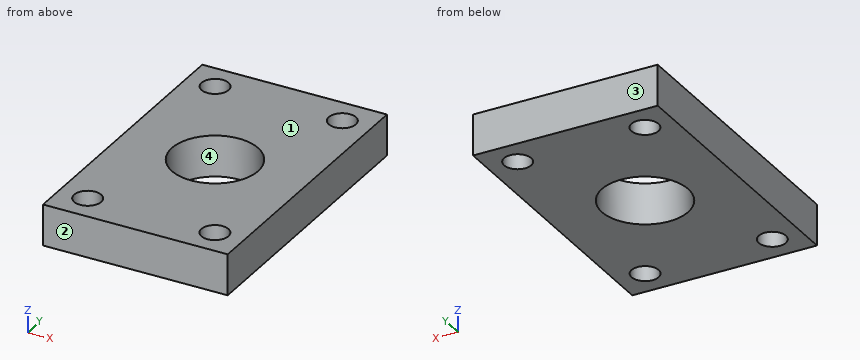
```python
from build123d import *

# Parameters (mm, degrees)
SCHIZZO1_W                   = 45
SCHIZZO1_H                   = 70
ESTRUSIONE_ESTRUSIONE1_DEPTH = 10
SCHIZZO2_R                   = 10.5
SCHIZZO2_R_2                 = 3.3
TAGLIO_ESTRUSIONE1_DEPTH     = 10


with BuildPart() as part:
    # Schizzo1 → Estrusione-Estrusione1 (new body)
    with BuildSketch(Plane.XY):
        with Locations((22.5, 35)):
            Rectangle(SCHIZZO1_W, SCHIZZO1_H)
    extrude(amount=-ESTRUSIONE_ESTRUSIONE1_DEPTH)

    # Schizzo2 → Taglio-Estrusione1 (cut)
    with BuildSketch(Plane.XY):
        with Locations((22.5, 35)):
            Circle(SCHIZZO2_R)
        with Locations((38, 7)):
            Circle(SCHIZZO2_R_2)
        with Locations(Location((38, 63, 0), (0, 0, 180))):
            Circle(SCHIZZO2_R_2)
        with Locations(Location((7, 7, 0), (0, 0, 180))):
            Circle(SCHIZZO2_R_2)
        with Locations((7, 63)):
            Circle(SCHIZZO2_R_2)
    extrude(amount=-TAGLIO_ESTRUSIONE1_DEPTH, mode=Mode.SUBTRACT)


solid = part.part
```
Can you work these out from the model? Positions are in its coordinate system, mm. Face numbers are marked on the shaded views. Give positions to 0.01 mm unless a question says otherwise; leave off trailing zeros. Loops run counter-clockwise (first coordinate to the right, second up) from the corner with the lowest first, then second, coordinate; pieces in that order, holes last. Notation, with made-up numbers: M -25,79.5 L 5,79.5 A31 cw 5,110.5 Z; hole C 32,-11 d7. An arc over 180 degrees is marked long. Use CSV: the item, a comma, the result in double quotes. Start each with the question number.
1. If I drill on L1, parallel to Y at x = 7, z = -6.25; L2, parallel to Y at x = 22.5, z = -4.5; L3, parallel to X at y = 7.5, z = -3.5, over which ranges is the centre line in solid material (lowest first)?
2. Imagine slicing it at C-C, the plane x = 39.5. Write out the boundary of the cut face in (y, z).
3. Imagine slicing it at A-A, the plane y = 7. Write out the boundary of the cut face in (x, z).
4. For P1, Ø1, axis at x = 22.5, y = 52, coming from the +Z side; P2, Ø12, axis at x = 25.5, y = 38, coming from the +Z side, each with a flat end and sliding along its axis, tell me the tip position at first contact or that it passes through.
5. If we mould it in two halves opening along Y, with no side actions, what happens to the marked faces 1, 2, 3 and 4? For each: released by +Y, released by -Y, zero draft, split by the parting line, or undercut.
6. Imagine slicing it at D-D, the plane y = 35. Write out the boundary of the cut face in (x, z), plus the area to 3 significant figures.
7. Imagine slicing it at B-B, the plane z = -3. Write out the boundary of the cut face in (x, y).
Response values:
1,L1,"0 to 3.7, 10.3 to 59.7, 66.3 to 70"
1,L2,"0 to 24.5, 45.5 to 70"
1,L3,"0 to 3.74, 10.26 to 34.74, 41.26 to 45"
2,outline,"M 0,-10 L 4.06,-10 L 4.06,0 L 0,0 Z; M 9.94,-10 L 60.06,-10 L 60.06,0 L 9.94,0 Z; M 65.94,-10 L 70,-10 L 70,0 L 65.94,0 Z"
3,outline,"M 0,-10 L 3.7,-10 L 3.7,0 L 0,0 Z; M 10.3,-10 L 34.7,-10 L 34.7,0 L 10.3,0 Z; M 41.3,-10 L 45,-10 L 45,0 L 41.3,0 Z"
4,P1,"z = 0"
4,P2,"through"
5,face 1,"zero draft"
5,face 2,"released by -Y"
5,face 3,"released by +Y"
5,face 4,"undercut"
6,outline,"M 0,-10 L 12,-10 L 12,0 L 0,0 Z; M 33,-10 L 45,-10 L 45,0 L 33,0 Z"
6,area,"240 mm^2"
7,outline,"M 0,0 L 45,0 L 45,70 L 0,70 Z; hole C 7,7 d6.6; hole C 7,63 d6.6; hole C 22.5,35 d21; hole C 38,7 d6.6; hole C 38,63 d6.6"
